Source: CAD feature listing. Evaluate the final solid. Frame: model axes, mm. A direction names the side the tool comes from. Give positions to 0.01 mm unless a question says otherwise; leave off trailing zeros. Write each loop counter-clockwise with the first axis right and the second up, starting at its lowest first coordinate (ties: lowest second). Pieces come first, ordered by that corner, then holes. Notation, with made-up numbers: (-23, 12.5) -> (20, 12.5) arc R5 ccw to (20, 21.5) -> close; hole circle Ø5 at (-32, 40.25). An arc over 180 degrees is marked (long way). Answer as a JSON object with one key per item and string values. Group by question number.
Item 1: Access query for faces 1 (the face through (51.261, 55.536, 1.479)), 2 (the face through (63, 20, 1)). Directions: +Z, -Z, +X, -X, +Y, -Y. A direction counts if a zero-diameter tool reaches every point of the face in a straight line with its end or side. Return the directions, or none.
Item 2: Ray query, probe 1 along Y at (x, z) = (50.5, 1.35); probe 2 along Y at (x, z) = (21, 0.35); probe 3 along Y at (x, z) = (5, 0.9). Return the intervals inside material, ascending. Write a range as from..to.
Item 3: Section query D-D on x = 34.5. Return the cut outline in (y, z), plus the area to 3 significant figures.
Item 4: Section query C-C on z = 2.05. Give the number of separate pieces and of enclosed holes in the cut face, plus the area to 3 significant figures.
Item 5: Section query A-A on x = 50.5. Return the cut outline in (y, z), plus the area to 3 significant figures.
Item 6: Pull-direction query (Y, two-part tool) for faces 3 (the face through (55.07, 61.5, 1.52)), 4 (the face through (70, 10, 1)), 5 (the face through (23.526, 11.352, 1.521)); classes: pulls with the +Y half, pulls with the -Y half, needs draft (parallel to the pull), parting line crosses it, or undercut.
Item 7: First-contact query: pin 1 Ø0.9 at (y, z) = (44.5, 2) entering from -X; pin 2 Ø1.5 at (y, z) = (36, 1.5) entering from +X; pin 3 Ø0.9 at (x, z) = (6, 1) entering from +Y. Flat tips, straight axial feed; report the tip coordinate or a pass-through.
Item 8: Section query B-B on y = 57. Return the cut outline in (x, z).
from build123d import *

# Parameters (mm, degrees)
SKETCH1_W           = 43
SKETCH1_H           = 43
SKETCH1_R           = 1.65
SKETCH1_W_2         = 70
SKETCH1_H_2         = 20
BOSS_EXTRUDE1_DEPTH = 3
FILLET1_R           = 5
SKETCH2_R           = 2
CUT_EXTRUDE1_DEPTH  = 3
SKETCH3_R           = 12.5
CUT_EXTRUDE2_DEPTH  = 3


with BuildPart() as part:
    # Sketch1 → Boss-Extrude1 (new body)
    with BuildSketch(Plane.XY):
        with Locations((35, 41.5)):
            Rectangle(SKETCH1_W, SKETCH1_H)
        with Locations((19.5, 26)):
            Circle(SKETCH1_R, mode=Mode.SUBTRACT)
        with Locations((50.5, 26)):
            Circle(SKETCH1_R, mode=Mode.SUBTRACT)
        with Locations((19.5, 57)):
            Circle(SKETCH1_R, mode=Mode.SUBTRACT)
        with Locations((50.5, 57)):
            Circle(SKETCH1_R, mode=Mode.SUBTRACT)
        with Locations((35, 10)):
            Rectangle(SKETCH1_W_2, SKETCH1_H_2)
    extrude(amount=BOSS_EXTRUDE1_DEPTH)

    # Fillet1
    fillet1_edges = [part.edges().sort_by_distance(p)[0] for p in [
        (56.5, 20, 1.5),
        (70, 20, 1.5),
        (70, 0, 1.5),
        (0, 0, 1.5),
        (0, 20, 1.5),
        (13.5, 20, 1.5),
        (13.5, 63, 1.5),
        (56.5, 63, 1.5),
    ]]
    fillet(fillet1_edges, radius=FILLET1_R)

    # Sketch2 → Cut-Extrude1 (cut)
    with BuildSketch(Plane.XY.offset(3)):
        with Locations((5, 10)):
            Circle(SKETCH2_R)
        with Locations((25, 10)):
            Circle(SKETCH2_R)
        with Locations((45, 10)):
            Circle(SKETCH2_R)
        with Locations((65, 10)):
            Circle(SKETCH2_R)
    extrude(amount=-CUT_EXTRUDE1_DEPTH, mode=Mode.SUBTRACT)

    # Sketch3 → Cut-Extrude2 (cut)
    with BuildSketch(Plane.XY.offset(3)):
        with Locations((34.5, 42)):
            Circle(SKETCH3_R)
    extrude(amount=-CUT_EXTRUDE2_DEPTH, mode=Mode.SUBTRACT)


solid = part.part
Worked answers:
{
 "1": {"face 1": "+Z, -Z", "face 2": "+Z, -Z, +X, +Y"},
 "2": {"probe 1": "0..24.35, 27.65..55.35, 58.65..63", "probe 2": "0..25.31, 26.69..56.31, 57.69..63", "probe 3": "0..8, 12..20"},
 "3": {"outline": "(0, 0) -> (29.5, 0) -> (29.5, 3) -> (0, 3) -> close; (54.5, 0) -> (63, 0) -> (63, 3) -> (54.5, 3) -> close", "area": "114 mm^2"},
 "4": {"separate pieces": "1", "enclosed holes": "9", "area": "2,650 mm^2"},
 "5": {"outline": "(0, 0) -> (24.35, 0) -> (24.35, 3) -> (0, 3) -> close; (27.65, 0) -> (55.35, 0) -> (55.35, 3) -> (27.65, 3) -> close; (58.65, 0) -> (63, 0) -> (63, 3) -> (58.65, 3) -> close", "area": "169 mm^2"},
 "6": {"face 3": "pulls with the +Y half", "face 4": "needs draft", "face 5": "undercut"},
 "7": {"pin 1": "x = 13.5", "pin 2": "x = 56.5", "pin 3": "y = 20"},
 "8": {"outline": "(13.5, 0) -> (17.85, 0) -> (17.85, 3) -> (13.5, 3) -> close; (21.15, 0) -> (48.85, 0) -> (48.85, 3) -> (21.15, 3) -> close; (52.15, 0) -> (56.5, 0) -> (56.5, 3) -> (52.15, 3) -> close"}
}
